The listing builds one solid part. Answer for the finished solid, in the listing's coordinates (mm). Face numbers are marked on the shaded views. A direction names the side the tool comes from. Give positions to 0.01 mm unless a question says otherwise; leave off trailing zeros. Write each loop counter-clockwise with the first axis right and the second up, starting at its lowest first coordinate (ties: lowest second). Pieces come first, ordered by that corner, then holes. Notation, with made-up numbers: (13, 12.25) - (27, 12.25) arc R30 cw to (27, 41.25) - close; hole circle Ø8 at (84.25, 88). An arc over 180 degrees is marked (long way). Answer as CSV lines item,"result". Start each with the question number.
(1) For the marked faces 1, 2, 3 and 4, determine the directions among +Z, -Z, +X, -X, +Y, -Y from which every point of the face is accessible in a straight line to the end or side of a thin tool.
(2) Straight lines are drawn through the part: probe 1 along X at (y, z) = (-44, 11); probe 2 along X at (y, z) = (-44, 3); probe 3 along Z at (x, y) = (70.5, -34.5) (3 decimals). For each, find the intervals that lie inside material, in ascending order.
(3) Each of these flat-tipped pins is pushed along its axis until it touches: pin 1 Ø4 at (y, z) = (-46.5, -3) entering from +X; pin 2 Ø2.5 at (y, z) = (-45, -2) entering from -X; pin 3 Ø9.5 at (x, y) = (43.5, -49) entering from +Z (3 decimals). Where does it stop, or does it pass through?
(4) Find section C-C (x = 26.5). Write down the section's boundary in (y, z) (1 decimal).
(5) Find section B-B (z = 14.5). Write down the section's boundary in (x, y) (3 decimals).
(6) For a pull along Y with two mould halves and no side action, classify the marked faces 5, 6 and 7 as pulls with the +Y half, pulls with the -Y half, needs draft (parallel to the pull), parting line crosses it, or undercut.
from build123d import *

# Parameters (mm, degrees)
F0_W           = 25.5704697987
F0_H           = 4.7625
F1_DEPTH       = 63.5
F3_DEPTH       = 15.875
F2_W           = 33.3017666123
F2_H           = 23.8125
F4_DEPTH       = 38.1
F6_D           = 12.7
F6_CBORE_D     = 19.05
F6_CBORE_DEPTH = 9.525
F8_DEPTH       = 50.8


with BuildPart() as f1:
    # F0 (on Front) → F1 (new body)
    with BuildSketch(Plane.XZ):
        Polygon((6.35, 15.875), (6.35, 0), (31.75, 0), (57.3204697987, 0), (82.55, 0), (82.55, 11.1125), (57.15, 11.1125), (57.15, 15.875), align=None)
        Polygon((0, 38.1), (0, 0), (6.35, 0), (6.35, 15.875), (6.35, 38.1), align=None)
        with Locations((44.5352348993, -2.38125)):
            Rectangle(F0_W, F0_H)
    extrude(amount=F1_DEPTH)

    # F2 (on Top) → F3 (join)
    with BuildSketch(Plane.XY):
        Polygon((82.55, -33.2294587481), (82.55, 0), (50.8, 0), (50.8, -10.5265528092), (39.6517666123, -23.8125), (6.35, -63.5), (41.275, -63.5), (57.15, -63.5), align=None)
    extrude(amount=F3_DEPTH)

    # F2 (on Top) → F4 (join)
    with BuildSketch(Plane.XY):
        with Locations((23.0008833062, -11.90625)):
            Rectangle(F2_W, F2_H)
        Polygon((50.8, -10.5265528092), (50.8, 0), (39.6517666123, 0), (39.6517666123, -23.8125), align=None)
        Polygon((6.35, -63.5), (39.6517666123, -23.8125), (6.35, -23.8125), align=None)
    extrude(amount=F4_DEPTH)

    # F6 (through all)
    with Locations(Plane.XY.offset(15.875)):
        with Locations((41.275, -44.45)):
            CounterBoreHole(F6_D / 2, F6_CBORE_D / 2, F6_CBORE_DEPTH)

    # F7 (on face) → F8 (cut)
    with BuildSketch(Plane.YZ.offset(50.8)):
        Polygon((-10.5265528092, 30.4293548129), (-10.5265528092, 38.1), (-23.8125, 38.1), align=None)
        Polygon((0, 24.3518467149), (0, 38.1), (-10.5265528092, 38.1), (-10.5265528092, 30.4293548129), align=None)
    extrude(amount=-F8_DEPTH, mode=Mode.SUBTRACT)


solid = f1.part
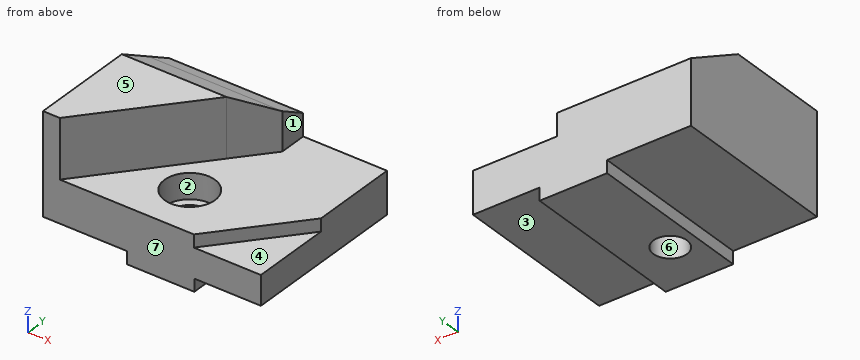
Result set:
1,face 1,"+Z, +X, +Y, -Y"
1,face 2,"+Z"
1,face 3,"-Z, +X, +Y, -Y"
1,face 4,"+Z, +X, -Y"
2,probe 1,"0 to 31.76, 50.79 to 82.55"
2,probe 2,"0 to 34.94, 47.61 to 82.55"
2,probe 3,"0 to 15.875"
3,pin 1,"x = 57.32"
3,pin 2,"x = 31.75"
3,pin 3,"z = 15.875"
4,outline,"(-63.5, 0) - (0, 0) - (0, 24.4) - (-23.8, 38.1) - (-39.5, 38.1) - (-39.5, 15.9) - (-63.5, 15.9) - close"
5,outline,"(0, -63.5) - (57.15, -63.5) - (82.55, -33.229) - (82.55, 0) - (0, 0) - close; hole circle Ø19.05 at (41.275, -44.45)"
6,face 5,"needs draft"
6,face 6,"undercut"
6,face 7,"pulls with the -Y half"
